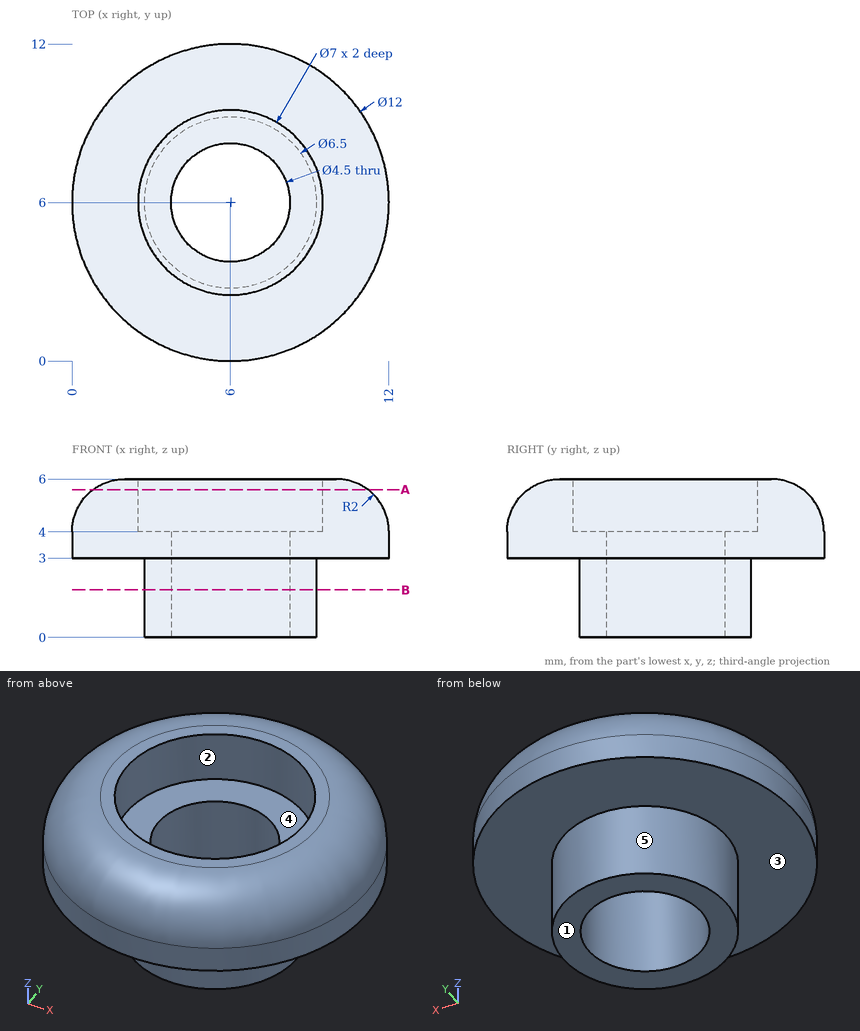
Geometry check sheet. Reference: drawing and pictorial views, mm from the part's lowest x, y, z. A direction names the side the tool comes from. Round coordinates to 2 decimals unless told otherwise and drop trailing zeros. Write each loop counter-clockwise with the first axis right and the second up, starting at its lowest first coordinate (ties: lowest second). Pieces come first, ordered by that corner, then holes.
Item 1: Mould release check, pull along Y, two halves, no side actions. Record for the marked faces 3, 4 and 5: +Y half, -Y half, draft (parallel to the pull), parting line (faces both ways), or undercut.
Determined:
face 3: draft
face 4: undercut
face 5: parting line
Item 2: Go/stop test with flat-tipped pins: pin 1 Ø2 at (x, z) = (9.5, 3) entering from -Y; pin 2 Ø4 at (x, y) = (6, 6) entering from +Z; pin 3 Ø2 at (x, z) = (2.5, 1.5) entering from +Y; pin 4 Ø5.5 at (x, y) = (6, 6) entering from +Z. Record where each tip stops, or that it passes through.
Determined:
pin 1: stops at y = 0.55
pin 2: passes through
pin 3: stops at y = 8.08
pin 4: stops at z = 4
Item 3: Section check B-B (z = 1.8). Record the boundary of the cut face in (x, y), plus the area to 3 significant figures.
Determined:
outline: circle Ø6.5 at (6, 6); hole circle Ø4.5 at (6, 6)
area: 17.3 mm2
Item 4: Section check A-A (z = 5.6). Record the boundary of the cut face in (x, y), plus the area to 3 significant figures.
Determined:
outline: circle Ø10.4 at (6, 6); hole circle Ø7 at (6, 6)
area: 46.5 mm2
Item 5: Access from +Z, -Z, +X, -X, +Y, -Y to the whole of each face (thin tool, end or side, straight path). Record for the marked faces 1 and 2.
Determined:
face 1: -Z, +X, -X, +Y, -Y
face 2: +Z
Item 6: Material ranges on line 1 along Y through (x, z) = (6, 2.2); line 2 along Z through (x, y) = (3.25, 3); line 3 along Y through (x, z) = (7.75, 0.6), recorded low to high.
Determined:
line 1: y = 2.75 to 3.75, 8.25 to 9.25
line 2: z = 3 to 6
line 3: y = 3.26 to 4.59, 7.41 to 8.74
